Can you work these out from the drawing? Everything is in mm from the part's minimum corner. A direction names the side the tool comes from. Round coordinates to 2 decimals unless told otherwise and drop trailing zeros. Loops run counter-clockwise (first coordinate to the right, second up) from the corner with the lowest first, then second, coordinate; pieces in that order, holes last. Notation, with made-up numbers: (26, 19) -> (56, 19) arc R26 cw to (56, 54) -> close; hole circle Ø3 at (2.25, 3). An arc over 180 degrees is marked (long way). One line per item, written item: value.
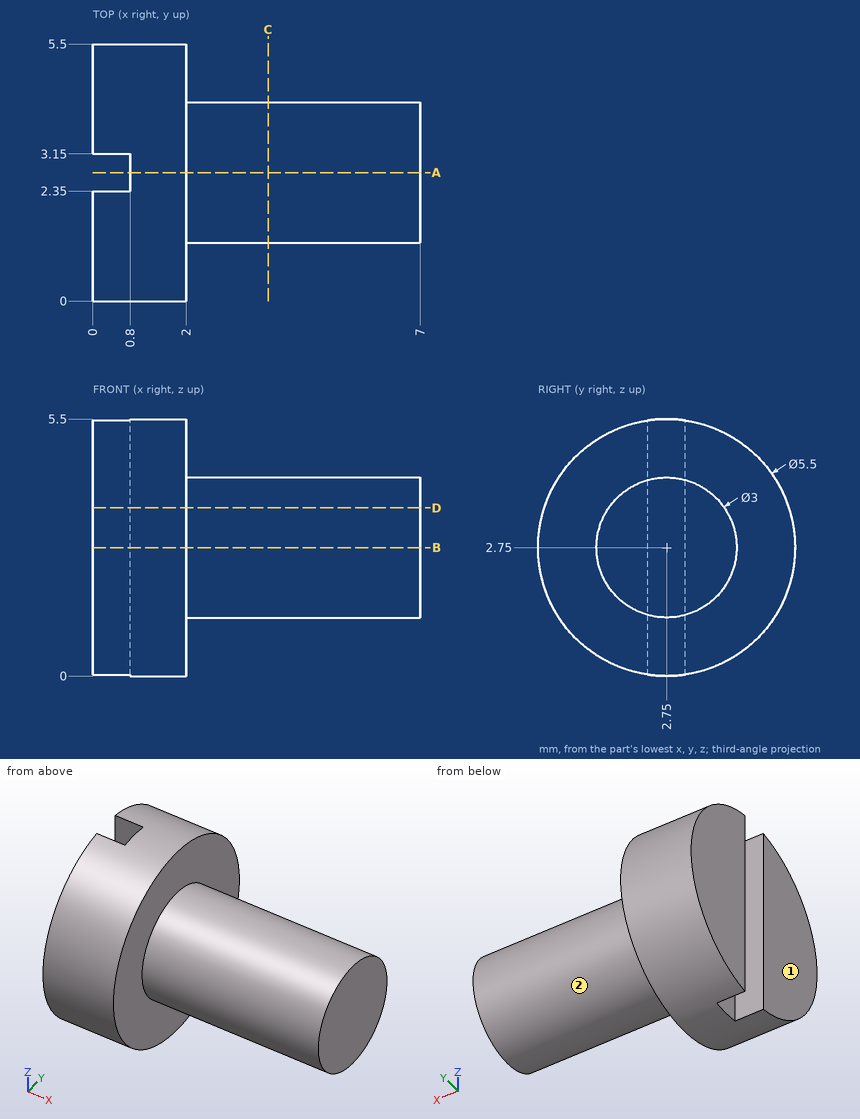
Item 1: Will these pins go through, and if not, where does the flat tip stop? pin 1 Ø0.6 at (x, z) = (0.5, 3.5) entering from +Y; pin 2 Ø1.5 at (x, z) = (4, 2) entering from -Y.
Output:
pin 1: stops at y = 5.46
pin 2: stops at y = 1.25
Item 2: I need wall thicknesses on line 1 (X direction, y = 1.25, z = 1.5); line 2 (X direction, y = 3, z = 2.75); line 3 (Z direction, x = 1.5, y = 0.9). Which ranges of each line are inside material? Lowest first, please. Write a range as from..to.
Output:
line 1: x = 0..2
line 2: x = 0.8..7
line 3: z = 0.72..4.78
Item 3: If we section it at B-B on z = 2.75: List the corners of the cut face in (x, y) for me.
Output:
outline: (0, 0) -> (2, 0) -> (2, 1.25) -> (7, 1.25) -> (7, 4.25) -> (2, 4.25) -> (2, 5.5) -> (0, 5.5) -> (0, 3.15) -> (0.8, 3.15) -> (0.8, 2.35) -> (0, 2.35) -> close
Item 4: If we section it at C-C on x = 3.75: List the corners of the cut face in (y, z) for me, plus the area to 3 significant figures.
Output:
outline: circle Ø3 at (2.75, 2.75)
area: 7.07 mm²
Item 5: For the marked faces 1 and 2, which set-ups out of +Z, -Z, +X, -X, +Y, -Y let a thin tool reach every point of the face, with its end or its side?
Output:
face 1: +Z, -Z, -X, +Y, -Y
face 2: +X
Item 6: If we section it at D-D on z = 3.6: List the corners of the cut face in (x, y) for me.
Output:
outline: (0, 0.13) -> (2, 0.13) -> (2, 1.51) -> (7, 1.51) -> (7, 3.99) -> (2, 3.99) -> (2, 5.37) -> (0, 5.37) -> (0, 3.15) -> (0.8, 3.15) -> (0.8, 2.35) -> (0, 2.35) -> close
Item 7: If we section it at A-A on y = 2.75: List the corners of the cut face in (x, z) for me.
Output:
outline: (0.8, 0) -> (2, 0) -> (2, 1.25) -> (7, 1.25) -> (7, 4.25) -> (2, 4.25) -> (2, 5.5) -> (0.8, 5.5) -> close
